CAD build for the part. Positions are in the model's coordinates, mm. A direction names the side the tool comes from. Coordinates: 2 decimals unless noted, no trailing zeros. Order: outer loops, then holes, each group sorted by start corner. A loop starts at its lowest first (then second) coordinate and runs counter-clockwise, first axis right, second up. Notation, with made-up numbers: (-14.75, 85.25) - (44.25, 85.25) arc R11 ccw to (44.25, 93.25) - close; hole circle Ø11 at (-9.5, 63.5). An arc over 180 degrees is marked (long way). Use one line per item in the form item = value.
```python
from build123d import *

# Parameters (mm, degrees)
CROQUIS1_R              = 1.5
SALIENTE_EXTRUIR1_DEPTH = 10
CROQUIS2_W              = 8
CROQUIS2_H              = 7.5
CROQUIS2_W_2            = 14
CROQUIS2_H_2            = 8
CROQUIS2_W_3            = 9
CORTAR_EXTRUIR1_DEPTH   = 2.6
REDONDEO1_R             = 1


with BuildPart() as part:
    # Croquis1 → Saliente-Extruir1 (new, symmetric)
    with BuildSketch(Plane(origin=(0, 0, 0), x_dir=(0, 0, -1), z_dir=(1, 0, 0))):
        with BuildLine():
            Line((-14, 4), (0, 4))
            Line((0, 4), (0, 16))
            ThreePointArc((0, 16), (4, 20), (8, 16))
            Line((8, 16), (8, 4))
            Line((8, 4), (14, 4))
            ThreePointArc((14, 4), (18, 0), (14, -4))
            Line((14, -4), (-14, -4))
            Line((-14, -4), (-34, -4))
            ThreePointArc((-34, -4), (-38, 0), (-34, 4))
            Line((-34, 4), (-14, 4))
        make_face()
        with Locations((14, 0)):
            Circle(CROQUIS1_R, mode=Mode.SUBTRACT)
        with Locations((4, 16)):
            Circle(CROQUIS1_R, mode=Mode.SUBTRACT)
        with Locations((-14, 0)):
            Circle(CROQUIS1_R, mode=Mode.SUBTRACT)
        with Locations((-34, 0)):
            Circle(CROQUIS1_R, mode=Mode.SUBTRACT)
    extrude(amount=SALIENTE_EXTRUIR1_DEPTH, both=True)

    # Croquis2 → Cortar-Extruir1 (cut, symmetric)
    with BuildSketch(Plane(origin=(0, 0, 0), x_dir=(0, 0, -1), z_dir=(1, 0, 0))):
        with Locations((4, 16.25)):
            Rectangle(CROQUIS2_W, CROQUIS2_H)
        with Locations((-14, 0)):
            Rectangle(CROQUIS2_W_2, CROQUIS2_H_2)
        with Locations((13.5, 0)):
            Rectangle(CROQUIS2_W_3, CROQUIS2_H_2)
        with Locations((-33.5, 0)):
            Rectangle(CROQUIS2_W_3, CROQUIS2_H_2)
    extrude(amount=CORTAR_EXTRUIR1_DEPTH, both=True, mode=Mode.SUBTRACT)

    # Redondeo1
    redondeo1_edges = [part.edges().sort_by_distance(p)[0] for p in [
        (2.6, 0, -9),
        (-2.6, 0, -9),
        (-2.6, 0, 7),
        (-2.6, 0, 21),
        (2.6, 0, 7),
        (2.6, 0, 21),
        (2.6, 0, 29),
        (-2.6, 0, 29),
    ]]
    fillet(redondeo1_edges, radius=REDONDEO1_R)


solid = part.part
```
Item 1: Cut at B-B, the plane z = -4. Write the cut outline in (x, y), plus the area to 3 significant figures.
Derived:
outline = (-10, -4) - (10, -4) - (10, 14.5) - (2.6, 14.5) - (2.6, 12.5) - (-2.6, 12.5) - (-2.6, 14.5) - (-10, 14.5) - close; (-10, 17.5) - (-2.6, 17.5) - (-2.6, 20) - (-10, 20) - close; (2.6, 17.5) - (10, 17.5) - (10, 20) - (2.6, 20) - close
area = 397 mm²
Item 2: 3-axis set-ups, long thin cutter, end or side, ignore diameter. For faces 1 (the face through (0, 0, -9)), 2 (the face through (2.315, 0.056, 20.699)), 3 (the face through (-2.315, 0.056, 29.301)): which of +Z, -Z, +X, -X, +Y, -Y reach the whole face in a straight line?
Derived:
face_1 = -Z, +Y, -Y
face_2 = +Y, -Y
face_3 = +Z, +Y, -Y
Item 3: Two-plate mould, pull along Y, no slides. Class faces 4 (the face through (6.248, 15.425, -5.386)), 5 (the face through (-6, 0, 38)), 6 (the face through (-2.6, 0, 32)): +Y half, -Y half, draft (parallel to the pull), parting line (faces both ways), or undercut.
Derived:
face_4 = undercut
face_5 = parting line
face_6 = draft
Item 4: Cut at A-A, the plane x = 5.5. Write the cut outline in (y, z), plus the area to 3 significant figures.
Derived:
outline = (-4, -14) arc R4 ccw to (4, -14) - (4, -8) - (16, -8) arc R4 ccw to (16, 0) - (4, 0) - (4, 34) arc R4 ccw to (-4, 34) - close; hole circle Ø3 at (0, -14); hole circle Ø3 at (0, 14); hole circle Ø3 at (0, 34); hole circle Ø3 at (16, -4)
area = 527 mm²
Item 5: Drill centre lines: line 1 (Z direction, x = 6, y = 0); line 2 (X direction, y = 1.5, z = -15.5); line 3 (Y direction, x = 5, z = 14). Where is each one in solid material? Low to high. Write a range as [from, to].
Derived:
line_1 = [-18, -15.5], [-12.5, 12.5], [15.5, 32.5], [35.5, 38]
line_2 = [-10, -2.6], [2.6, 10]
line_3 = [-4, -1.5], [1.5, 4]
Item 6: Cut at D-D, the plane y = 2.5. Write the cut outline in (x, z).
Derived:
outline = (-10, -17.12) - (-2.6, -17.12) - (-2.6, -10) arc R1 cw to (-1.6, -9) - (1.6, -9) arc R1 cw to (2.6, -10) - (2.6, -17.12) - (10, -17.12) - (10, 37.12) - (2.6, 37.12) - (2.6, 30) arc R1 cw to (1.6, 29) - (-1.6, 29) arc R1 cw to (-2.6, 30) - (-2.6, 37.12) - (-10, 37.12) - close; hole (-2.6, 8) arc R1 ccw to (-1.6, 7) - (1.6, 7) arc R1 ccw to (2.6, 8) - (2.6, 20) arc R1 ccw to (1.6, 21) - (-1.6, 21) arc R1 ccw to (-2.6, 20) - close
Item 7: Cut at C-C, the plane z = 16.5. Write the cut outline in (x, y).
Derived:
outline = (-10, -4) - (-2.6, -4) - (-2.6, 4) - (-10, 4) - close; (2.6, -4) - (10, -4) - (10, 4) - (2.6, 4) - close
Item 8: Drop flat-ended pins along their axis: pin 1 (9.5 mm diameter, centred on x = 0.5, y = 10, fed in from +Z); pin 2 (4 mm diameter, centred on y = 16, z = -4, fed in from -X); pin 3 (8 mm diameter, centred on x = -6, y = 5, fed in from -Z); pin 4 (1 mm diameter, centred on x = 0.5, y = -1.5, fed in from -Z). Give the stop position or say it passes through.
Derived:
pin_1 = 0
pin_2 = -10
pin_3 = -17.87
pin_4 = -9
